Input: dimensioned drawing with shaded views. Units: mm. Origin: part minimum x, y, z. Give positions to 0.01 mm unless a question says otherwise; leave off trailing zeros. Write each loop counter-clockwise with the first axis right and the second up, starting at its lowest first coordinate (ties: lowest second). Pieces come first, ordered by that corner, then holes.
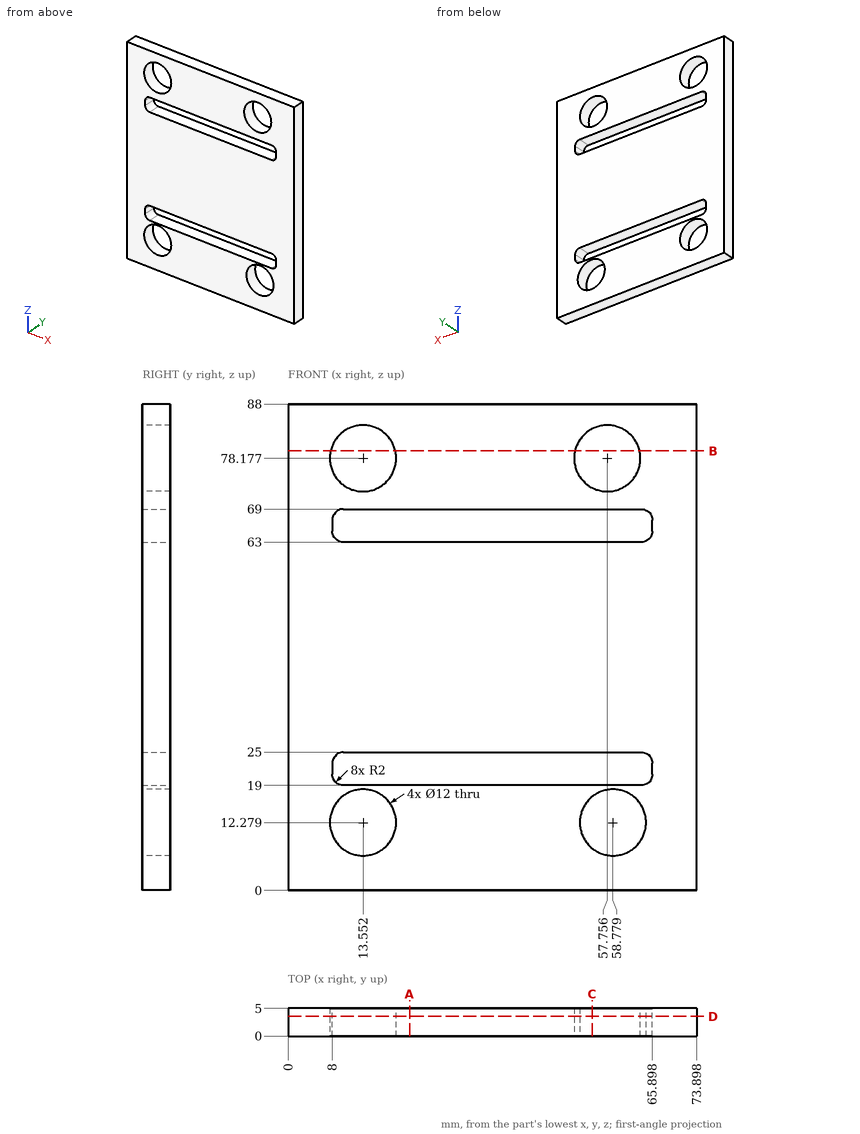
Item 1: Section A-A, the plane x = 22. Return the cut outline in (y, z).
Found:
outline: (0, 0) - (5, 0) - (5, 19) - (0, 19) - close; (0, 25) - (5, 25) - (5, 63) - (0, 63) - close; (0, 69) - (5, 69) - (5, 88) - (0, 88) - close
Item 2: Line query: L1, parallel to Z at x = 47, y = 3.5; L2, parallel to X at y = 1.4, z = 21.5; L3, parallel to X at y = 4.7, z = 79 (1 decimal). Output: solid intervals per line, ascending.
Found:
L1: z = 0 to 19, 25 to 63, 69 to 88
L2: x = 0 to 8, 65.9 to 73.9
L3: x = 0 to 7.6, 19.5 to 51.8, 63.7 to 73.9
Item 3: Pin query (flat end, axial travel): pin 1 Ø3 at (x, z) = (44.5, 36.5) entering from -Y. Return the tip coordinate at first contact, or that it passes through.
Found:
pin 1: stops at y = 0
Item 4: Section D-D, the plane y = 3.55. Return the cut outline in (x, z).
Found:
outline: (0, 0) - (73.9, 0) - (73.9, 88) - (0, 88) - close; hole circle Ø12 at (13.55, 12.28); hole circle Ø12 at (13.55, 78.18); hole (8, 21) arc R2 ccw to (10, 19) - (63.9, 19) arc R2 ccw to (65.9, 21) - (65.9, 23) arc R2 ccw to (63.9, 25) - (10, 25) arc R2 ccw to (8, 23) - close; hole (8, 65) arc R2 ccw to (10, 63) - (63.9, 63) arc R2 ccw to (65.9, 65) - (65.9, 67) arc R2 ccw to (63.9, 69) - (10, 69) arc R2 ccw to (8, 67) - close; hole circle Ø12 at (57.76, 78.18); hole circle Ø12 at (58.78, 12.28)
Item 5: Section B-B, the plane z = 79.5. Return the cut outline in (x, y).
Found:
outline: (0, 0) - (7.7, 0) - (7.7, 5) - (0, 5) - close; (19.4, 0) - (51.9, 0) - (51.9, 5) - (19.4, 5) - close; (63.61, 0) - (73.9, 0) - (73.9, 5) - (63.61, 5) - close
Item 6: Section C-C, the plane x = 55. Return the cut outline in (y, z).
Found:
outline: (0, 0) - (5, 0) - (5, 7.62) - (0, 7.62) - close; (0, 16.94) - (5, 16.94) - (5, 19) - (0, 19) - close; (0, 25) - (5, 25) - (5, 63) - (0, 63) - close; (0, 69) - (5, 69) - (5, 72.85) - (0, 72.85) - close; (0, 83.51) - (5, 83.51) - (5, 88) - (0, 88) - close
